Can you work these out from the model? Positions are in its coordinate system, mm. A direction names the side the tool comes from. Give positions to 0.01 mm unless a question says otherwise; leave off trailing zeros. Loops run counter-clockwise (first coordinate to the right, second up) from the corner with the lowest first, then second, coordinate; pieces in that order, holes last. Notation, with made-up numbers: (7.25, 63.25) -> (18.25, 63.25) arc R17 ccw to (18.25, 71.25) -> close; hole circle Ø11 at (62, 23.25). An arc over 180 degrees is marked (long way). Return JSON: item names as keys, results as strings. Group by question number.
Q1. I need wall thicknesses on line 1 along Y through (x, z) = (-2, 2.55); line 2 along X through (y, z) = (14, 2.85); line 3 along Y through (x, z) = (-11, 1.15). Which ranges of each line are inside material? Lowest first, please. Write a range as [from, to].
Q2. Suppose I cut it at C-C, the plane y = -11.5. Please give me the cut outline in (x, z), and give its area (3 significant figures).
Q3. Suppose I cut it at B-B, the plane x = -15.5. Please give me the cut outline in (y, z).
Q4. Will these pins go through, and if not, where does the flat tip stop? pin 1 (1.5 mm diameter, centred on y = 15.5, z = 0.5, fed in from +X); pin 2 (10 mm diameter, centred on x = -1.5, y = -19.5, fed in from -Z); pin 3 (1 mm diameter, centred on y = 0.5, z = 1, fed in from +X); pin 4 (1 mm diameter, centred on y = 20, z = 1, fed in from +X).
Q5. Suppose I cut it at A-A, the plane y = 0.5. Please give me the cut outline in (x, z).
Q6. Which directions (+Z, -Z, +X, -X, +Y, -Y) give clear straight access to the entire face, cutting with the end or side of a thin tool? Please do faces 1 (the cylindrical face through (-8.1, 25.23, 1.58)), 2 (the flat face through (-3.5, 0, 2)).
Q7. Thinking about a two-plate mould opening in X: for faces 3 (the flat face through (-1.8, 3, 1.6)), 4 (the flat face through (3, -5, 3.2)), 5 (the flat face through (-1.726, -3.045, 1.578)), 6 (the cylindrical face through (13.503, -0.124, 1.578)), which applies, pulls with the +X half, pulls with the -X half, needs draft (parallel to the pull), parting line crosses it, or undercut?
```python
from build123d import *

# Parameters (mm, degrees)
F1_DEPTH = 3.2
F2_R     = 5


with BuildPart() as f1:
    # F0 (on Top) → F1 (new body)
    with BuildSketch(Plane.XY):
        with BuildLine():
            ThreePointArc((-12.36068, 17.013016), (-10.923029, 7.936045), (-20, 6.498394))
            ThreePointArc((-20, 6.498394), (-26.498394, 0), (-20, -6.498394))
            ThreePointArc((-20, -6.498394), (-10.923029, -7.936045), (-12.36068, -17.013016))
            ThreePointArc((-12.36068, -17.013016), (-8.188454, -25.20147), (0, -21.029244))
            ThreePointArc((0, -21.029244), (4.172226, -12.84079), (12.36068, -17.013016))
            ThreePointArc((12.36068, -17.013016), (21.437651, -15.575365), (20, -6.498394))
            ThreePointArc((20, -6.498394), (13.501606, 0), (20, 6.498394))
            ThreePointArc((20, 6.498394), (21.437651, 15.575365), (12.36068, 17.013016))
            ThreePointArc((12.36068, 17.013016), (4.172226, 12.84079), (0, 21.029244))
            ThreePointArc((0, 21.029244), (-8.188454, 25.20147), (-12.36068, 17.013016))
        make_face()
        Polygon((0, 4.041452), (3.5, 2.020726), (3.5, -2.020726), (0, -4.041452), (-3.5, -2.020726), (-3.5, 2.020726), align=None, mode=Mode.SUBTRACT)
    extrude(amount=F1_DEPTH)

    # F2
    f2_edges = [f1.edges().sort_by_distance(p)[0] for p in [
        (-12.36068, 17.013016, 1.6),
        (-20, 6.498394, 1.6),
        (0, 21.029244, 1.6),
        (12.36068, 17.013016, 1.6),
        (20, 6.498394, 1.6),
        (20, -6.498394, 1.6),
        (12.36068, -17.013016, 1.6),
        (0, -21.029244, 1.6),
        (-12.36068, -17.013016, 1.6),
        (-20, -6.498394, 1.6),
    ]]
    fillet(f2_edges, radius=F2_R)


solid = f1.part
```
Ans:
{
 "1": {"line 1": "y = [-23.99, -2.89], [2.89, 23.99]", "line 2": "x = [-10.08, 2.06], [10.31, 22.28]", "line 3": "y = [-23.38, -15.68], [-7.83, 7.83], [15.68, 23.38]"},
 "2": {"outline": "(-9.69, 0) -> (22.67, 0) -> (22.67, 3.2) -> (-9.69, 3.2) -> close", "area": "104 mm^2"},
 "3": {"outline": "(-5.29, 0) -> (5.29, 0) -> (5.29, 3.2) -> (-5.29, 3.2) -> close"},
 "4": {"pin 1": "stops at x = 21.95", "pin 2": "stops at z = 0", "pin 3": "stops at x = 13.58", "pin 4": "stops at x = -0.26"},
 "5": {"outline": "(-26.48, 0) -> (-3.5, 0) -> (-3.5, 3.2) -> (-26.48, 3.2) -> close; (3.5, 0) -> (13.52, 0) -> (13.52, 3.2) -> (3.5, 3.2) -> close"},
 "6": {"face 1": "+Z, -Z, +Y", "face 2": "+Z, -Z"},
 "7": {"face 3": "undercut", "face 4": "needs draft", "face 5": "undercut", "face 6": "pulls with the +X half"}
}
